Source: CAD feature listing. Evaluate the final solid. Frame: model axes, mm. A direction names the side the tool comes from. Coordinates: 2 decimals unless noted, no trailing zeros. Loops run counter-clockwise (first coordinate to the right, second up) from the corner with the lowest first, then second, coordinate; pieces in that order, holes last.
Item 1: Pin query (flat end, axial travel): pin 1 Ø5 at (x, z) = (14.79, 14) entering from -Y; pin 2 Ø10 at (x, y) = (26, -55) entering from -Z; pin 3 Ø1 at (x, y) = (41.5, -56) entering from +Z; pin 4 Ø12 at (y, z) = (-59, -4) entering from +X. Return the tip coordinate at first contact, or that it passes through.
Item 2: Section query D-D, the plane y = -46. State how many separate pieces and enclosed holes the cut face has, then the cut area to 3 significant figures.
Item 3: Section query A-A, the plane z = 14. Return the cut outline in (x, y).
Item 4: Line query: probe 1 along Y at (x, z) = (26, 14.5); probe 2 along Z at (x, y) = (16, -55.5); probe 3 along X at (y, z) = (-47.25, -17). Output: solid intervals per line, ascending.
Item 5: Section query C-C, the plane z = -22.5. Return the cut outline in (x, y), then the cut area to 3 significant figures.
Item 6: Section query B-B, the plane x = 38. Return the cut outline in (y, z).
Item 7: Reachability of faces 1 (the cylindrical face through (18.979, -46.968, -42.993)), 2 (the flat face through (27, -59, 0)), 3 (the flat face through (27, -49.433, 14)) from +Z, -Z, +X, -X, +Y, -Y: full face, straight path, thin tool, end or side. Return the list, or none.
Item 8: Pull-direction query (X, two-part tool) for faces 4 (the cylindrical face through (7.932, -46.898, 22.797)), 5 (the flat face through (27, -49.433, -17)), 6 (the cylindrical face through (46.286, -68.531, 1.972)), 7 (the cylindrical face through (35.767, -46.968, -42.338)); classes: +X half, -X half, draft (parallel to the pull), parting line (faces both ways), or undercut.
```python
from build123d import *

# Parameters (mm, degrees)
SKETCH1_R           = 1.73
SKETCH1_R_2         = 1.75
BOSS_EXTRUDE1_DEPTH = 4
SKETCH2_W           = 40.35
SKETCH2_H           = 5
BOSS_EXTRUDE2_DEPTH = 20
FILLET1_R           = 4
SKETCH3_R           = 1.85
CUT_EXTRUDE1_DEPTH  = 65.55458112
SKETCH4_W           = 42.335046752
SKETCH4_H           = 40.534615669
CUT_EXTRUDE2_DEPTH  = 87.274206212
SKETCH5_W           = 40.35
SKETCH5_H           = 5
BOSS_EXTRUDE3_DEPTH = 44
SKETCH7_R           = 8.132834804
SKETCH7_R_2         = 1.25
CUT_EXTRUDE3_DEPTH  = 10


with BuildPart() as part:
    # Sketch1 → Boss-Extrude1 (new body)
    with BuildSketch(Plane.XY):
        with BuildLine():
            Line((44.141212793, -69.433023223), (9.791212793, -69.433023223))
            ThreePointArc((9.791212793, -69.433023223), (7.669892449, -68.554343566), (6.791212793, -66.433023223))
            Line((6.791212793, -66.433023223), (6.791212793, -12.433023223))
            ThreePointArc((6.791212793, -12.433023223), (8.255678887, -8.897489317), (11.791212793, -7.433023223))
            Line((11.791212793, -7.433023223), (42.141212793, -7.433023223))
            ThreePointArc((42.141212793, -7.433023223), (45.676746699, -8.897489317), (47.141212793, -12.433023223))
            Line((47.141212793, -12.433023223), (47.141212793, -66.433023223))
            ThreePointArc((47.141212793, -66.433023223), (46.262533136, -68.554343566), (44.141212793, -69.433023223))
        make_face()
        with Locations((12.021212793, -14.663023223)):
            Circle(SKETCH1_R, mode=Mode.SUBTRACT)
        with Locations((41.911212793, -14.663023223)):
            Circle(SKETCH1_R, mode=Mode.SUBTRACT)
        with Locations((12.021212793, -38.723023223)):
            Circle(SKETCH1_R_2, mode=Mode.SUBTRACT)
        with Locations((41.911212793, -38.723023223)):
            Circle(SKETCH1_R_2, mode=Mode.SUBTRACT)
        with Locations((41.911212793, -59.433023223)):
            Circle(SKETCH1_R, mode=Mode.SUBTRACT)
        with Locations((12.021212793, -59.433023223)):
            Circle(SKETCH1_R, mode=Mode.SUBTRACT)
    extrude(amount=BOSS_EXTRUDE1_DEPTH)

    # Sketch2 → Boss-Extrude2 (add)
    with BuildSketch(Plane.XY.offset(4)):
        with Locations((26.966212793, -46.933023223)):
            Rectangle(SKETCH2_W, SKETCH2_H)
    extrude(amount=BOSS_EXTRUDE2_DEPTH)

    # Fillet1
    fillet1_edges = [part.edges().sort_by_distance(p)[0] for p in [
        (6.791212793, -46.933023223, 24),
        (47.141212793, -46.933023223, 24),
    ]]
    fillet(fillet1_edges, radius=FILLET1_R)

    # Sketch3 → Cut-Extrude1 (cut, through all)
    with BuildSketch(Plane(origin=(0, -44.433023223, 0), x_dir=(1, 0, 0), z_dir=(0, 1, 0))):
        with Locations(Location((39.141212793, -14, 0), (0, 0, 180))):
            Circle(SKETCH3_R)
        with Locations(Location((14.791212793, -14, 0), (0, 0, 180))):
            Circle(SKETCH3_R)
    extrude(amount=-CUT_EXTRUDE1_DEPTH, mode=Mode.SUBTRACT)

    # Sketch4 → Cut-Extrude2 (cut, through all)
    with BuildSketch(Plane.XY.offset(4)):
        with Locations((27.958736169, -24.165715389)):
            Rectangle(SKETCH4_W, SKETCH4_H)
    extrude(amount=-CUT_EXTRUDE2_DEPTH, mode=Mode.SUBTRACT)

    # Sketch5 → Boss-Extrude3 (add)
    with BuildSketch(Plane(origin=(0, 0, 0), x_dir=(-1, 0, 0), z_dir=(0, 0, -1))):
        with Locations((-26.966212793, -46.933023223)):
            Rectangle(SKETCH5_W, SKETCH5_H)
    extrude(amount=BOSS_EXTRUDE3_DEPTH)

    # Sketch7 → Cut-Extrude3 (cut)
    with BuildSketch(Plane.XZ.offset(49.433023223)):
        with Locations((20.836658571, -24.545339617)):
            Circle(SKETCH7_R)
        with Locations((18.309091346, -14.16226231)):
            Circle(SKETCH7_R_2)
        with Locations((10.808955155, -28.238854835)):
            Circle(SKETCH7_R_2)
        with Locations((19.249573785, -41.772459571)):
            Circle(SKETCH7_R_2)
        with Locations((35.190328606, -41.229471782)):
            Circle(SKETCH7_R_2)
        with Locations((42.690464797, -27.152879257)):
            Circle(SKETCH7_R_2)
        with Locations((34.249846167, -13.619274521)):
            Circle(SKETCH7_R_2)
        with BuildLine():
            Line((6.791212793, -24.680714066), (4.582649711, -44))
            Line((4.582649711, -44), (32.677324571, -51.00034411))
            Line((32.677324571, -51.00034411), (44.945122218, -48.614200906))
            Line((44.945122218, -48.614200906), (51.549779096, -38.819864159))
            Line((51.549779096, -38.819864159), (47.141212793, -27.190260187))
            add(Edge.make_bspline(
                [(26.749709976, -47.324288879), (47.770737556, -45.874846264), (47.141212793, -27.190260187)],
                knots=[0, 0, 0, 1, 1, 1], degree=2))
            add(Edge.make_bspline(
                [(6.791212793, -24.680714066), (6.595021886, -44.867895731), (26.749709976, -47.324288879)],
                knots=[0, 0, 0, 1, 1, 1], degree=2))
        make_face()
    extrude(amount=-CUT_EXTRUDE3_DEPTH, mode=Mode.SUBTRACT)


solid = part.part
```
Verdict:
1. pin 1: stops at y = -49.43
1. pin 2: stops at z = 0
1. pin 3: stops at z = 4
1. pin 4: stops at x = 47.14
2. separate pieces: 1
2. enclosed holes: 9
2. area: 2,400 mm2
3. outline: (6.79, -49.43) - (12.94, -49.43) - (12.94, -44.43) - (6.79, -44.43) - close; (16.64, -49.43) - (37.29, -49.43) - (37.29, -44.43) - (16.64, -44.43) - close; (40.99, -49.43) - (47.14, -49.43) - (47.14, -44.43) - (40.99, -44.43) - close
4. probe 1: y = -49.43 to -44.43
4. probe 2: z = 0 to 4
4. probe 3: x = 6.79 to 17.8, 23.87 to 47.14
5. outline: (6.79, -49.43) - (12.97, -49.43) - (12.97, -44.43) - (6.79, -44.43) - close; (28.71, -49.43) - (47.14, -49.43) - (47.14, -44.43) - (28.71, -44.43) - close
5. area: 123 mm2
6. outline: (-69.43, 0) - (-49.43, 0) - (-49.43, -44) - (-44.43, -44) - (-44.43, 12.54) - (-49.43, 12.54) - (-49.43, 4) - (-69.43, 4) - close; (-49.43, 15.46) - (-44.43, 15.46) - (-44.43, 24) - (-49.43, 24) - close
7. face 1: +Y, -Y
7. face 2: -Z, +X, -X, -Y
7. face 3: +Z, +X, -X, -Y
8. face 4: -X half
8. face 5: draft
8. face 6: +X half
8. face 7: undercut
